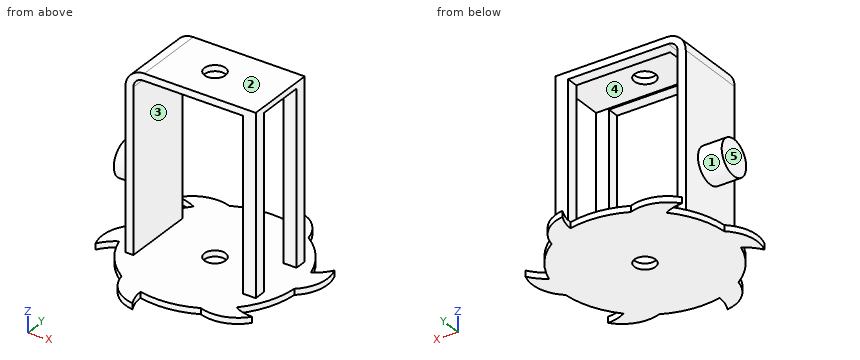
from build123d import *

# Parameters (mm, degrees)
SKETCH1_R           = 35
BOSS_EXTRUDE1_DEPTH = 2.5
SKETCH11_R          = 4.45
CUT_EXTRUDE5_DEPTH  = 10
BOSS_EXTRUDE4_START = 75
SKETCH5_W           = 55
SKETCH5_H           = 30
SKETCH5_R           = 4.45
BOSS_EXTRUDE4_DEPTH = 75
SKETCH6_W           = 72.5
SKETCH6_H           = 20
CUT_EXTRUDE2_DEPTH  = 45
SKETCH7_R           = 7.5
BOSS_EXTRUDE5_DEPTH = 10
CUT_EXTRUDE3_DEPTH  = 30
FILLET1_R           = 8


with BuildPart() as part:
    # Sketch1 → Boss-Extrude1 (new body)
    with BuildSketch(Plane.XY):
        with BuildLine():
            ThreePointArc((-33.502769568, -10.1274099), (-34.767453022, -4.027928789), (-34.930842804, 2.199140974))
            ThreePointArc((-34.930842804, 2.199140974), (-40.093982991, -6.182304711), (-39.373214245, -16))
            ThreePointArc((-39.373214245, -16), (-36.802059341, -12.69977052), (-33.502769568, -10.1274099))
        make_face()
        Circle(SKETCH1_R)
        with BuildLine():
            ThreePointArc((-25.521979032, 23.950544593), (-20.872015167, 28.095533148), (-15.560909452, 31.350567731))
            ThreePointArc((-15.560909452, 31.350567731), (-25.401024429, 31.631255454), (-33.543013583, 26.098203765))
            ThreePointArc((-33.543013583, 26.098203765), (-29.399353563, 25.521633041), (-25.521979032, 23.950544593))
        make_face()
        with BuildLine():
            ThreePointArc((7.980790536, 34.077954493), (13.895437855, 32.123461937), (19.369933352, 29.151426756))
            ThreePointArc((19.369933352, 29.151426756), (14.692958562, 37.813560165), (5.830200662, 42.098203765))
            ThreePointArc((5.830200662, 42.098203765), (7.402705778, 38.221403561), (7.980790536, 34.077954493))
        make_face()
        with BuildLine():
            ThreePointArc((34.930842804, -2.199140974), (40.093982991, 6.182304711), (39.373214245, 16))
            ThreePointArc((39.373214245, 16), (36.802059341, 12.69977052), (33.502769568, 10.1274099))
            ThreePointArc((33.502769568, 10.1274099), (34.623669179, 5.11874326), (35, 0))
            ThreePointArc((35, 0), (34.982706429, -1.100114056), (34.930842804, -2.199140974))
        make_face()
        with BuildLine():
            ThreePointArc((33.543013583, -26.098203765), (29.399353563, -25.521633041), (25.521979032, -23.950544593))
            ThreePointArc((25.521979032, -23.950544593), (20.872015167, -28.095533148), (15.560909452, -31.350567731))
            ThreePointArc((15.560909452, -31.350567731), (25.401024429, -31.631255454), (33.543013583, -26.098203765))
        make_face()
        with BuildLine():
            ThreePointArc((-5.830200662, -42.098203765), (-7.402705778, -38.221403561), (-7.980790536, -34.077954493))
            ThreePointArc((-7.980790536, -34.077954493), (-13.895437855, -32.123461937), (-19.369933352, -29.151426756))
            ThreePointArc((-19.369933352, -29.151426756), (-14.692958562, -37.813560165), (-5.830200662, -42.098203765))
        make_face()
    extrude(amount=BOSS_EXTRUDE1_DEPTH)

    # Sketch11 → Cut-Extrude5 (cut)
    with BuildSketch(Plane.XY.offset(2.5)):
        Circle(SKETCH11_R)
    extrude(amount=-CUT_EXTRUDE5_DEPTH, mode=Mode.SUBTRACT)

    # Sketch5 → Boss-Extrude4 (add)
    with BuildSketch(Plane.XY.offset(2.5).offset(BOSS_EXTRUDE4_START)):
        Rectangle(SKETCH5_W, SKETCH5_H)
        Circle(SKETCH5_R, mode=Mode.SUBTRACT)
    extrude(amount=-BOSS_EXTRUDE4_DEPTH)

    # Sketch6 → Cut-Extrude2 (cut)
    with BuildSketch(Plane(origin=(27.5, 0, 0), x_dir=(0, 0, -1), z_dir=(1, 0, 0))):
        with Locations((-38.75, 0)):
            Rectangle(SKETCH6_W, SKETCH6_H)
    extrude(amount=-CUT_EXTRUDE2_DEPTH, mode=Mode.SUBTRACT)

    # Sketch7 → Boss-Extrude5 (add)
    with BuildSketch(Plane.ZY.offset(27.5)):
        with Locations(Location((30, 0, 0), (0, 0, 270))):
            Circle(SKETCH7_R)
    extrude(amount=BOSS_EXTRUDE5_DEPTH)

    # Sketch8 → Cut-Extrude3 (cut)
    with BuildSketch(Plane.XZ.offset(15)):
        with BuildLine():
            Line((-24.082664687, 70.5), (-24.082664687, 2.5))
            Line((-24.082664687, 2.5), (22.085730974, 2.5))
            Line((22.085730974, 2.5), (22.085730974, 74.5))
            Line((22.085730974, 74.5), (-20.082664687, 74.5))
            ThreePointArc((-20.082664687, 74.5), (-22.911091812, 73.328427125), (-24.082664687, 70.5))
        make_face()
    extrude(amount=-CUT_EXTRUDE3_DEPTH, mode=Mode.SUBTRACT)

    # Fillet1
    fillet1_edges = [part.edges().sort_by_distance(p)[0] for p in [
        (-27.5, 0, 77.5),
    ]]
    fillet(fillet1_edges, radius=FILLET1_R)


solid = part.part
Geometry check sheet. Reference: the model listing, model coordinates, mm. Face numbers are marked on the shaded views. A direction names the side the tool comes from. Give positions to 0.01 mm unless a question says otherwise; leave off trailing zeros. Order: outer loops, then holes, each group sorted by start corner. A loop starts at its lowest first (then second) coordinate and runs counter-clockwise, first axis right, second up. Notation, with made-up numbers: (53.5, 80.25) - (101.5, 80.25) arc R20 ccw to (101.5, 106.25) - close; hole circle Ø9 at (-34, 75.25). An arc over 180 degrees is marked (long way). Use one line per item in the form item = value.
1) Sectioned sample at D-D (y = 0). Record the boundary of the cut face in (x, z), and give its area (3 significant figures).
Working result:
outline = (-37.5, 22.5) - (-27.5, 22.5) - (-27.5, 2.5) - (-37.06, 2.5) - (-37.06, 0) - (-4.45, 0) - (-4.45, 2.5) - (-24.08, 2.5) - (-24.08, 70.5) arc R4 cw to (-20.08, 74.5) - (-17.5, 74.5) - (-17.5, 75) - (-4.45, 75) - (-4.45, 77.5) - (-19.5, 77.5) arc R8 ccw to (-27.5, 69.5) - (-27.5, 37.5) - (-37.5, 37.5) - close; (4.45, 0) - (37.06, 0) - (37.06, 2.5) - (4.45, 2.5) - close; (4.45, 75) - (27.5, 75) - (27.5, 77.5) - (4.45, 77.5) - close
area = 669 mm^2
2) Draft check along X on the marked faces 3, 4 and 5. Enter one of: released by +X, released by -X, zero draft, split by the parting line, or undercut.
Working result:
face_3 = undercut
face_4 = zero draft
face_5 = released by -X
3) Depth check by flat-ended pin: pin 1 Ø4 at (x, z) = (-25, 21) entering from +Y; pin 2 Ø24 at (y, z) = (-2.5, 35) entering from -X; pin 3 Ø2.5 at (y, z) = (11.5, 35) entering from -X; pin 4 Ø10 at (x, y) = (30.5, 2.5) entering from -Z. Enter the tip coordinate at first touch or a pass-through.
Working result:
pin_1 = 15
pin_2 = -37.5
pin_3 = -27.5
pin_4 = 0
4) Sectioned sample at A-A (z = 7.5). Record the boundary of the cut face in (x, y).
Working result:
outline = (-27.5, -15) - (-24.08, -15) - (-24.08, 15) - (-27.5, 15) - close; (22.09, -15) - (27.5, -15) - (27.5, -10) - (22.09, -10) - close; (22.09, 10) - (27.5, 10) - (27.5, 15) - (22.09, 15) - close
5) Material ranges on probe 1 along Z at (x, y) = (-5.5, 1.5); probe 2 along Y at (x, z) = (0, 76.2); probe 3 along Y at (x, z) = (0, 1.2), recorded low to high. Write a range as from..to.
Working result:
probe_1 = 0..2.5, 75..77.5
probe_2 = -15..-4.45, 4.45..15
probe_3 = -35..-4.45, 4.45..35
6) Sectioned sample at B-B (x = 0). Record the boundary of the cut face in (y, z).
Working result:
outline = (-35, 0) - (-4.45, 0) - (-4.45, 2.5) - (-35, 2.5) - close; (-15, 74.5) - (-10, 74.5) - (-10, 75) - (-4.45, 75) - (-4.45, 77.5) - (-15, 77.5) - close; (4.45, 0) - (35, 0) - (35, 2.5) - (4.45, 2.5) - close; (4.45, 75) - (10, 75) - (10, 74.5) - (15, 74.5) - (15, 77.5) - (4.45, 77.5) - close
7) Sectioned sample at C-C (x = -30). Record the boundary of the cut face in (y, z).
Working result:
outline = (-18.03, 0) - (18.03, 0) - (18.03, 2.5) - (-18.03, 2.5) - close; circle Ø15 at (0, 30); (25.67, 0) - (29.44, 0) - (29.44, 2.5) - (25.67, 2.5) - close
8) Access from +Z, -Z, +X, -X, +Y, -Y to the whole of each face (thin tool, end or side, straight path). Record for the marked faces 1 and 2.
Working result:
face_1 = -X
face_2 = +Z, +X, -X, +Y, -Y
